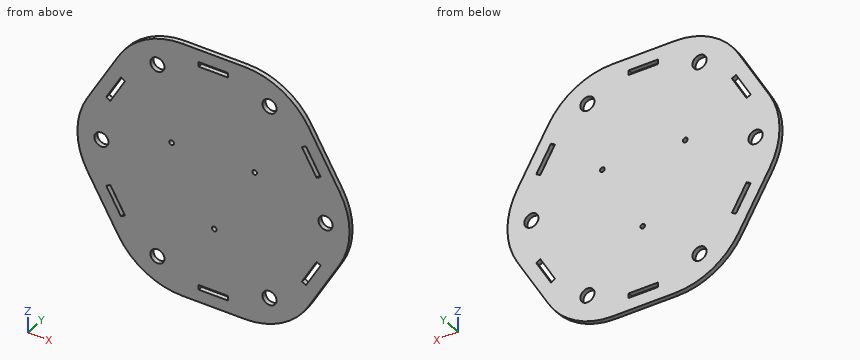
from build123d import *

# Parameters (mm, degrees)
SKETCH1_W           = 40
SKETCH1_H           = 6.35
BOSS_EXTRUDE1_DEPTH = 6.35
SKETCH2_R           = 3.2
CUT_EXTRUDE1_DEPTH  = 6.35
SKETCH3_R           = 9.5885
CUT_EXTRUDE2_DEPTH  = 254.16323495


with BuildPart() as part:
    # Sketch1 → Boss-Extrude1 (new body)
    with BuildSketch(Plane(origin=(0, 0, 0), x_dir=(1, 0, 0), z_dir=(0, 1, 0))):
        with BuildLine():
            Line((171.132486541, 50), (128.867513459, 123.205080757))
            ThreePointArc((128.867513459, 123.205080757), (92.264973081, 159.807621135), (42.264973081, 173.205080757))
            Line((42.264973081, 173.205080757), (-42.264973081, 173.205080757))
            ThreePointArc((-42.264973081, 173.205080757), (-92.264973081, 159.807621135), (-128.867513459, 123.205080757))
            Line((-128.867513459, 123.205080757), (-171.132486541, 50))
            ThreePointArc((-171.132486541, 50), (-184.529946162, 0), (-171.132486541, -50))
            Line((-171.132486541, -50), (-128.867513459, -123.205080757))
            ThreePointArc((-128.867513459, -123.205080757), (-92.264973081, -159.807621135), (-42.264973081, -173.205080757))
            Line((-42.264973081, -173.205080757), (42.264973081, -173.205080757))
            ThreePointArc((42.264973081, -173.205080757), (92.264973081, -159.807621135), (128.867513459, -123.205080757))
            Line((128.867513459, -123.205080757), (171.132486541, -50))
            ThreePointArc((171.132486541, -50), (184.529946162, 0), (171.132486541, 50))
        make_face()
        with Locations((0, -153.175)):
            Rectangle(SKETCH1_W, SKETCH1_H, mode=Mode.SUBTRACT)
        Polygon((-139.903810568, -57.679491924), (-145.403071882, -60.854491924), (-125.403071882, -95.495508076), (-119.903810568, -92.320508076), align=None, mode=Mode.SUBTRACT)
        Polygon((-119.903810568, 92.320508076), (-125.403071882, 95.495508076), (-145.403071882, 60.854491924), (-139.903810568, 57.679491924), align=None, mode=Mode.SUBTRACT)
        with Locations((0, 153.175)):
            Rectangle(SKETCH1_W, SKETCH1_H, mode=Mode.SUBTRACT)
        Polygon((139.903810568, 57.679491924), (145.403071882, 60.854491924), (125.403071882, 95.495508076), (119.903810568, 92.320508076), align=None, mode=Mode.SUBTRACT)
        Polygon((119.903810568, -92.320508076), (125.403071882, -95.495508076), (145.403071882, -60.854491924), (139.903810568, -57.679491924), align=None, mode=Mode.SUBTRACT)
    extrude(amount=BOSS_EXTRUDE1_DEPTH)

    # Sketch2 → Cut-Extrude1 (cut)
    with BuildSketch(Plane(origin=(0, 6.35, 0), x_dir=(1, 0, 0), z_dir=(0, 1, 0))):
        with Locations(Location((55.794244464, -33.346698257, 0), (0, 0, 270))):
            Circle(SKETCH2_R)
        with Locations(Location((-56.776210055, -31.645883963, 0), (0, 0, 270))):
            Circle(SKETCH2_R)
        with Locations(Location((0.981965591, 64.99258222, 0), (0, 0, 270))):
            Circle(SKETCH2_R)
    extrude(amount=-CUT_EXTRUDE1_DEPTH, mode=Mode.SUBTRACT)

    # Sketch3 → Cut-Extrude2 (cut, through all)
    with BuildSketch(Plane(origin=(0, 6.35, 0), x_dir=(1, 0, 0), z_dir=(0, 1, 0))):
        with Locations(Location((76, 131.635861375, 0), (0, 0, 270))):
            Circle(SKETCH3_R)
        with Locations(Location((152, 0, 0), (0, 0, 270))):
            Circle(SKETCH3_R)
        with Locations(Location((76, -131.635861375, 0), (0, 0, 270))):
            Circle(SKETCH3_R)
        with Locations(Location((-76, -131.635861375, 0), (0, 0, 270))):
            Circle(SKETCH3_R)
        with Locations(Location((-152, 0, 0), (0, 0, 270))):
            Circle(SKETCH3_R)
        with Locations(Location((-76, 131.635861375, 0), (0, 0, 270))):
            Circle(SKETCH3_R)
    extrude(amount=-CUT_EXTRUDE2_DEPTH, mode=Mode.SUBTRACT)


solid = part.part
Build history of the part. All positions in model axes, mm. Coordinates: 2 decimals unless noted, no trailing zeros. Order: outer loops, then holes, each group sorted by start corner. A loop starts at its lowest first (then second) coordinate and runs counter-clockwise, first axis right, second up. Notation, with made-up numbers: (86.5, 67) - (118.5, 67) arc R20 cw to (118.5, 83) - close; hole circle Ø3 at (54, 2.25). An arc over 180 degrees is marked (long way). Write item = value, one per line. Start each with the question number.
1) Saw through at B-B on x = -76. Write the cut outline in (y, z), then the cut area to 3 significant figures.
2) Saw through at D-D on y = 1.25. Count the separate pieces of the cut face and the enclosed holes in it, then the cut area to 3 significant figures.
3) Saw through at C-C on x = 152. Write the cut outline in (y, z).
4) Saw through at A-A on z = 0. Write the cut outline in (x, y).
5) Flat gauge pins, fed straight in: pin 1 Ø15.5 at (x, z) = (-152, 0) entering from -Y; pin 2 Ø22 at (x, z) = (76, -131.64) entering from +Y; pin 3 Ø1.9 at (y, z) = (3, -153) entering from +X; pin 4 Ø1.5 at (x, y) = (114.5, 4.5) entering from -Z. Where does each tip first touch, or does it go through?
6) Wall check: line 1 along Z through (x, y) = (-6, 6); line 2 along X through (y, z) = (0.5, 129); line 3 along X through (y, z) = (4.5, 0). Give the ranges that are in metal, low to high. Write a range as from..to.
From the geometry:
q1.outline = (0, -167.34) - (6.35, -167.34) - (6.35, -141.22) - (0, -141.22) - close; (0, -122.05) - (6.35, -122.05) - (6.35, 122.05) - (0, 122.05) - close; (0, 141.22) - (6.35, 141.22) - (6.35, 167.34) - (0, 167.34) - close
q1.area = 1,880 mm^2
q2.separate_pieces = 1
q2.enclosed_holes = 15
q2.area = 97,300 mm^2
q3.outline = (0, -83.14) - (6.35, -83.14) - (6.35, -9.59) - (0, -9.59) - close; (0, 9.59) - (6.35, 9.59) - (6.35, 83.14) - (0, 83.14) - close
q4.outline = (-184.53, 0) - (-161.59, 0) - (-161.59, 6.35) - (-184.53, 6.35) - close; (-142.41, 0) - (142.41, 0) - (142.41, 6.35) - (-142.41, 6.35) - close; (161.59, 0) - (184.53, 0) - (184.53, 6.35) - (161.59, 6.35) - close
q5.pin_1 = through
q5.pin_2 = 6.35
q5.pin_3 = 103.77
q5.pin_4 = -143.13
q6.line_1 = -173.21..-156.35, -150..150, 156.35..173.21
q6.line_2 = -125.25..-85.22, -66.78..66.78, 85.22..125.25
q6.line_3 = -184.53..-161.59, -142.41..142.41, 161.59..184.53
